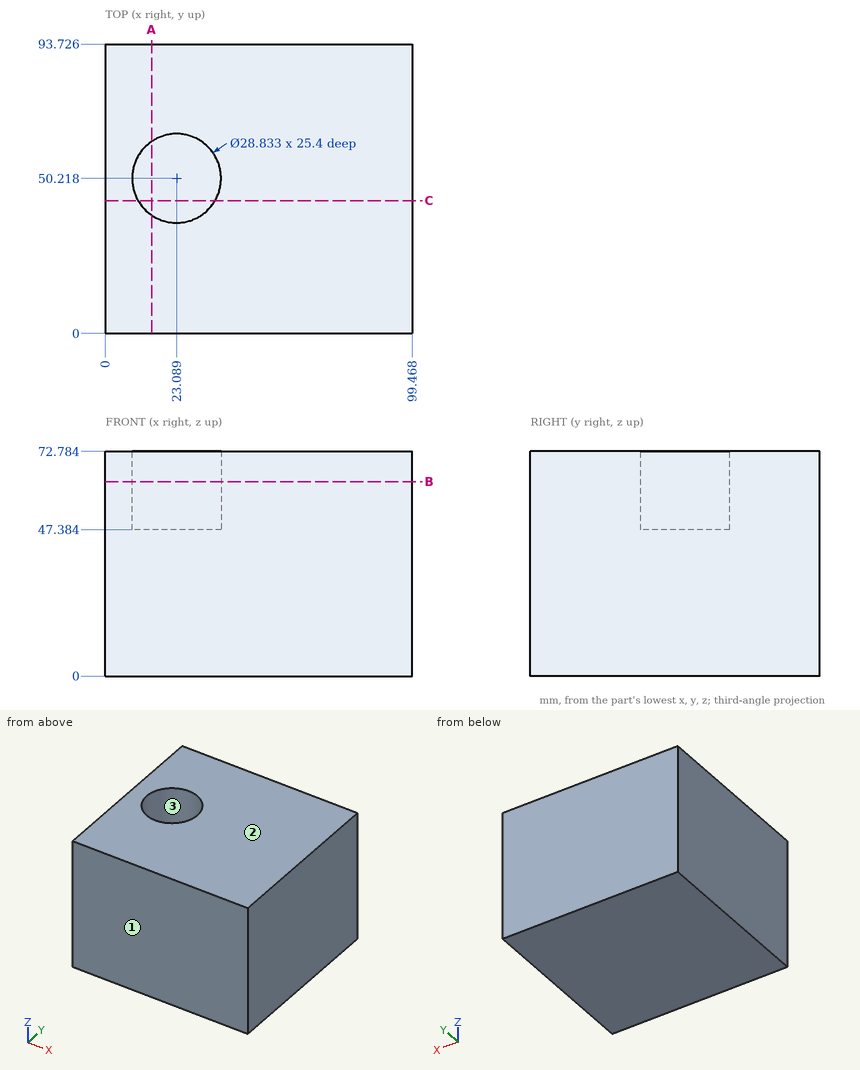
Part print with two shaded views. Sizes in mm from the minimum x, y, z corner. Coordinates: 2 decimals unless noted, no trailing zeros. Write each loop counter-clockwise with the first axis right and the second up, starting at its lowest first coordinate (ties: lowest second). Pieces come first, ordered by that corner, then holes. Notation, with made-up numbers: (45.25, 6) - (74.25, 6) arc R9 cw to (74.25, 10) - close; hole circle Ø8 at (63.5, 27). An arc over 180 degrees is marked (long way). Put each result on its own line as item: value.
1. Two-plate mould, pull along Y, no slides. Class the marked faces 1, 2 and 3: +Y half, -Y half, draft (parallel to the pull), parting line (faces both ways), or undercut.
Final values:
face 1: -Y half
face 2: draft
face 3: undercut
2. Band-saw the part on A-A (x = 15). Write the cut outline in (y, z) (1 decimal), then the cut area to 3 significant figures.
Final values:
outline: (0, 0) - (93.7, 0) - (93.7, 72.8) - (62.2, 72.8) - (62.2, 47.4) - (38.3, 47.4) - (38.3, 72.8) - (0, 72.8) - close
area: 6,220 mm²
3. Flat gauge pin, fed straight in: pin 1 Ø1 at (x, z) = (37, 36) entering from -Y. Where does the tip first touch, or does it go through?
Final values:
pin 1: stops at y = 0
4. Band-saw the part on B-B (z = 63). Write the cut outline in (x, y), then the cut area to 3 significant figures.
Final values:
outline: (0, 0) - (99.47, 0) - (99.47, 93.73) - (0, 93.73) - close; hole circle Ø28.83 at (23.09, 50.22)
area: 8,670 mm²
5. Band-saw the part on C-C (y = 43). Write the cut outline in (x, z), then the cut area to 3 significant figures.
Final values:
outline: (0, 0) - (99.47, 0) - (99.47, 72.78) - (35.57, 72.78) - (35.57, 47.38) - (10.61, 47.38) - (10.61, 72.78) - (0, 72.78) - close
area: 6,610 mm²
6. Probe line 1 along Y through (x, z) = (24, 61.5) (1 decimal); line 2 along Z through (x, y) = (22, 47); line 3 along Y through (x, z) = (26, 55.5) (1 decimal). List the from-to ranges inside material, lowest first. Write a range as [from, to].
Final values:
line 1: y = [0, 35.8], [64.6, 93.7]
line 2: z = [0, 47.38]
line 3: y = [0, 36.1], [64.3, 93.7]
